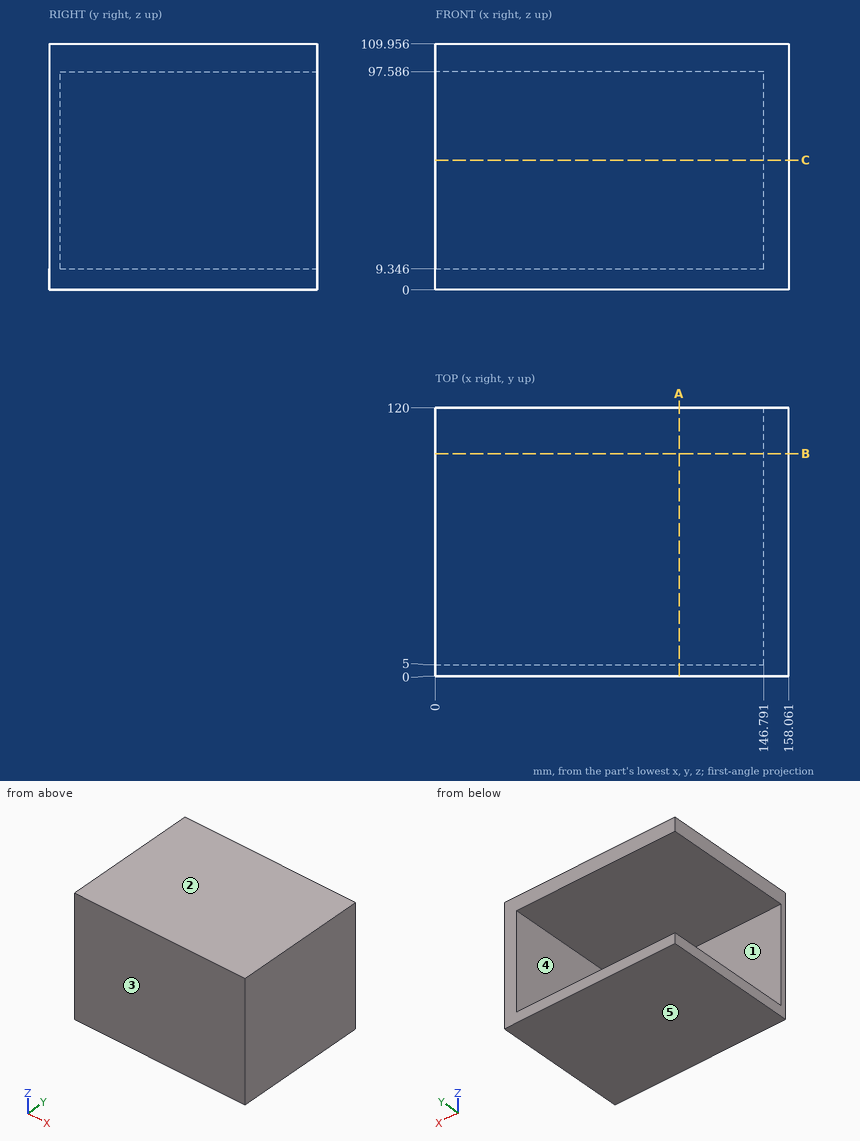
Design review of the part shown in the three views and the two pictorial views. Dimensions are in mm from the part's minimum x, y and z. A direction names the side the tool comes from. Round coordinates to 2 decimals unless told otherwise and drop trailing zeros. Loops run counter-clockwise (first coordinate to the right, second up) from the corner with the lowest first, then second, coordinate; pieces in that order, holes last.
1) Clearance check with a flat-ended pin moving along its axis: P1, Ø5, axis at y = 105, z = 92, coming from the -X side. State where the tip first meets the part, or that it passes through.
Values follow:
P1: stops at x = 146.79
2) The part is to be moulded in two halves that separate along Y. For the marked faces 1, 2 and 3, say which applies: pulls with the +Y half, pulls with the -Y half, needs draft (parallel to the pull), parting line crosses it, or undercut.
Values follow:
face 1: pulls with the +Y half
face 2: needs draft
face 3: pulls with the -Y half
3) Consider section B-B on y = 99.5. State the section outline as (x, z) points (1 decimal).
Values follow:
outline: (0, 0) - (158.1, 0) - (158.1, 110) - (0, 110) - (0, 97.6) - (146.8, 97.6) - (146.8, 9.3) - (0, 9.3) - close
4) Consider section A-A on x = 109. State the section outline as (y, z) points (1 decimal).
Values follow:
outline: (0, 0) - (120, 0) - (120, 9.3) - (5, 9.3) - (5, 97.6) - (120, 97.6) - (120, 110) - (0, 110) - close
5) Consider section C-C on z = 58. State the section outline as (x, y) points.
Values follow:
outline: (0, 0) - (158.06, 0) - (158.06, 120) - (146.79, 120) - (146.79, 5) - (0, 5) - close
6) Wall thickness on line 1 along Z through (x, y) = (69, 56.5) (1 decimal); line 2 along Y through (x, z) = (135, 44); line 3 along X through (y, z) = (68.5, 53): over which ranges is each line inside the solid? List them lowest first.
Values follow:
line 1: z = 0 to 9.3, 97.6 to 110
line 2: y = 0 to 5
line 3: x = 146.79 to 158.06
7) Tool access review of the marked faces 4 and 5: name each direction out of +Z, -Z, +X, -X, +Y, -Y from which nothing blocks a thin tool from reaching the whole face with its end or side.
Values follow:
face 4: -X, +Y
face 5: -Z, +X, -X, +Y, -Y
